```python
from build123d import *

# Parameters (mm, degrees)
SKETCH1_R               = 35
BOSS_EXTRUDE1_DEPTH     = 10
SKETCH2_R               = 23.5
BOSS_EXTRUDE2_DEPTH     = 13
BOSS_EXTRUDE3_DEPTH     = 4
SKETCH4_R               = 1.5
CUT_EXTRUDE1_DEPTH      = 4
MIRROR2_COPY_1_SKETCH_R = 1.5
MIRROR2_COPY_1_DEPTH    = 4
BOSS_EXTRUDE4_DEPTH     = 3
FILLET1_R               = 2
FILLET1_OF_MIRROR3_R    = 2
SKETCH6_W               = 14
SKETCH6_H               = 26
BOSS_EXTRUDE5_DEPTH     = 3
SKETCH7_R               = 10
CUT_EXTRUDE3_DEPTH      = 10


with BuildPart() as part:
    # Sketch1 → Boss-Extrude1 (new body)
    with BuildSketch(Plane.XY):
        Circle(SKETCH1_R)
    extrude(amount=BOSS_EXTRUDE1_DEPTH)

    # Sketch2 → Boss-Extrude2 (add)
    with BuildSketch(Plane.XY.offset(10)):
        with Locations(Location((0, 0, 0), (0, 0, 180))):
            Circle(SKETCH2_R)
    extrude(amount=BOSS_EXTRUDE2_DEPTH)

    # Sketch3 → Boss-Extrude3 (add)
    with BuildSketch(Plane(origin=(0, 13, 0), x_dir=(1, 0, 0), z_dir=(0, 1, 0))):
        Polygon((35, -23), (-35, -23), (-43.809511096, -30.392057511), (-43.809511096, -35.392057511), (-23.422250333, -52.499000499), (23.422250333, -52.499000499), (43.809511096, -35.392057511), (43.809511096, -30.392057511), align=None)
    boss_extrude3 = extrude(amount=-BOSS_EXTRUDE3_DEPTH)

    # Sketch4 → Cut-Extrude1 (cut)
    with BuildSketch(Plane(origin=(0, 13, 0), x_dir=(1, 0, 0), z_dir=(0, 1, 0))):
        with Locations(Location((-40.809511096, -32.892057511, 0), (0, 0, 270))):
            Circle(SKETCH4_R)
    cut_extrude1 = extrude(amount=-CUT_EXTRUDE1_DEPTH, mode=Mode.SUBTRACT)

    # Mirror1: Cut-Extrude1 across plane
    add(cut_extrude1.mirror(Plane(origin=(0, 0, 0), x_dir=(0, 0, 1), z_dir=(1, 0, 0))), mode=Mode.SUBTRACT)

    # Mirror2: Boss-Extrude3, Cut-Extrude1 across plane
    add(boss_extrude3.mirror(Plane.ZX))
    add(cut_extrude1.mirror(Plane.ZX), mode=Mode.SUBTRACT)

    # Mirror2 copy 1 sketch → Mirror2 copy 1 (cut)
    with BuildSketch(Plane(origin=(0, -13, 0), x_dir=(-1, 0, 0), z_dir=(0, -1, 0))):
        with Locations(Location((-40.809511096, -32.892057511, 0), (0, 0, 270))):
            Circle(MIRROR2_COPY_1_SKETCH_R)
    extrude(amount=-MIRROR2_COPY_1_DEPTH, mode=Mode.SUBTRACT)

    # Sketch5 → Boss-Extrude4 (add)
    with BuildSketch(Plane.XY.offset(23)):
        Polygon((0, -13), (2, -13), (2, -22), (0, -22), (-2, -22), (-2, -13), align=None)
    boss_extrude4 = extrude(amount=BOSS_EXTRUDE4_DEPTH)

    # Fillet1
    fillet1_edges = [part.edges().sort_by_distance(p)[0] for p in [
        (-2, -22, 24.5),
        (2, -22, 24.5),
    ]]
    fillet(fillet1_edges, radius=FILLET1_R - 0.0001)  # a hair under: the kernel refuses the full size

    # Mirror3: Boss-Extrude4 across plane
    add(boss_extrude4.mirror(Plane.ZX))

    # Fillet1 of Mirror3
    fillet1_of_mirror3_edges = [part.edges().sort_by_distance(p)[0] for p in [
        (-2, 22, 24.5),
        (2, 22, 24.5),
    ]]
    fillet(fillet1_of_mirror3_edges, radius=FILLET1_OF_MIRROR3_R - 0.0001)  # a hair under: the kernel refuses the full size

    # Sketch6 → Boss-Extrude5 (add)
    with BuildSketch(Plane.XY.offset(52.499000499)):
        Rectangle(SKETCH6_W, SKETCH6_H)
    extrude(amount=BOSS_EXTRUDE5_DEPTH)

    # Sketch7 → Cut-Extrude3 (cut)
    with BuildSketch(Plane(origin=(0, 0, 0), x_dir=(-1, 0, 0), z_dir=(0, 0, -1))):
        Circle(SKETCH7_R)
    extrude(amount=-CUT_EXTRUDE3_DEPTH, mode=Mode.SUBTRACT)


solid = part.part
```
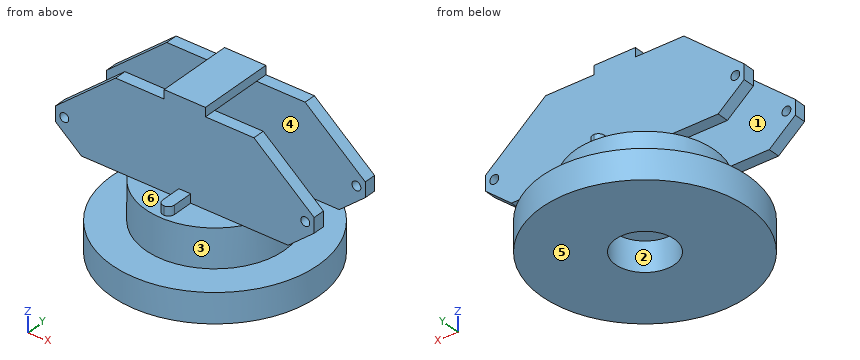
Geometry check sheet. Reference: the model listing, model coordinates, mm. Face numbers are marked on the shaded views. A direction names the side the tool comes from. Give positions to 0.01 mm unless a question says otherwise; leave off trailing zeros. Write each loop counter-clockwise with the first axis right and the second up, starting at its lowest first coordinate (ties: lowest second). Pieces come first, ordered by that corner, then holes.
1) Section check B-B, the plane z = 37.5. Record the boundary of the cut face in (x, y), and give its area (3 significant figures).
2) Release check for a two-part mould opening along X. For the marked faces 1, 2 and 3 record: pulls with the +X half, pulls with the -X half, needs draft (parallel to the pull), parting line crosses it, or undercut.
3) Material ranges on L1, parallel to Y at x = 21.5, z = 26; L2, parallel to Y at x = 0, z = 2; L3, parallel to Z at x = -5.5, y = 26, recorded low to high.
4) Access from +Z, -Z, +X, -X, +Y, -Y to the whole of each face (thin tool, end or side, straight path). Record for the marked faces 4, 5 and 6.
5) Section check D-D, the plane z = 21. Record the boundary of the cut face in (x, y).
6) Section check A-A, the plane y = 0. Record the boundary of the cut face in (x, z).
7) Gauge pin test, flat ends, axial feed: pin 1 (12 mm diameter, centred on x = -17.5, y = -27.5, fed in from -Z); pin 2 (3 mm diameter, centred on x = -12, y = -10, fed in from +Z); pin 3 (1 mm diameter, centred on x = 19.5, y = 4, fed in from +Z); pin 4 (4 mm diameter, centred on x = 10, z = 12.5, fed in from -Y). Record the tip position at first contact, or that the pin passes through.
8) Section check C-C, the plane x = 16. Record the boundary of the cut face in (y, z).
Computed:
1. outline: (-41.3, -13) - (41.3, -13) - (41.3, -9) - (-41.3, -9) - close; (-41.3, 9) - (41.3, 9) - (41.3, 13) - (-41.3, 13) - close
1. area: 661 mm2
2. face 1: needs draft
2. face 2: undercut
2. face 3: parting line crosses it
3. L1: y = -13 to -9, 9 to 13
3. L2: y = -35 to -10, 10 to 35
3. L3: z = 0 to 10
4. face 4: +X, -X
4. face 5: -Z, +X, -X, +Y, -Y
4. face 6: +Z, -Y
5. outline: circle Ø47 at (0, 0)
6. outline: (-35, 0) - (-10, 0) - (-10, 10) - (10, 10) - (10, 0) - (35, 0) - (35, 10) - (23.5, 10) - (23.5, 23) - (-23.5, 23) - (-23.5, 10) - (-35, 10) - close; (-7, 52.5) - (7, 52.5) - (7, 55.5) - (-7, 55.5) - close
7. pin 1: stops at z = 0
7. pin 2: stops at z = 52.5
7. pin 3: stops at z = 23
7. pin 4: stops at y = -22.1
8. outline: (-31.13, 0) - (31.13, 0) - (31.13, 10) - (17.21, 10) - (17.21, 23) - (13, 23) - (13, 52.5) - (9, 52.5) - (9, 23) - (-9, 23) - (-9, 52.5) - (-13, 52.5) - (-13, 23) - (-17.21, 23) - (-17.21, 10) - (-31.13, 10) - close
